Work out the finished part from the listing and answer in its coordinate system (mm). A direction names the side the tool comes from. Coordinates: 2 decimals unless noted, no trailing zeros. Loops run counter-clockwise (first coordinate to the right, second up) from the corner with the lowest first, then second, coordinate; pieces in that order, holes last. Notation, with made-up numbers: M 61,-24 L 89,-24 A19 ccw 89,-9 Z; hole C -8,50.5 d7. An arc over 180 degrees is marked long. Write each question's results on one line, items separated by ' | '.
```python
from build123d import *

# Parameters (mm, degrees)
F1_DEPTH = 63.5
F2_DEPTH = 12.7
F3_DEPTH = 25.4
F0_W     = 30.6498706341
F0_H     = 39.8745834827
F5_R     = 5.08


with BuildPart() as f1:
    # F0 (on Front) → F1 (new body, symmetric)
    with BuildSketch(Plane.XZ):
        Polygon((37.4401323497, 22.1690796316), (-51.7774410546, 22.1690796316), (-51.7774410546, -22.1690796316), (51.7774410546, -22.1690796316), (51.7774410546, 22.1690796316), align=None)
    extrude(amount=F1_DEPTH, both=True)

    # F0 (on Front) → F2 (join, symmetric)
    with BuildSketch(Plane.XZ):
        with BuildLine():
            Line((37.4401323497, 51.2318972406), (37.4401323497, 22.1690796316))
            Line((37.4401323497, 22.1690796316), (51.7774410546, 22.1690796316))
            Line((51.7774410546, 22.1690796316), (51.7774410546, 51.2318972406))
            ThreePointArc((51.7774410546, 51.2318972406), (57.0358954685, 63.9269292039), (69.7309274318, 69.1853836179))
            Line((69.7309274318, 69.1853836179), (80.344311893, 69.1853836179))
            Line((80.344311893, 69.1853836179), (80.344311893, 83.5226923227))
            Line((80.344311893, 83.5226923227), (69.7309274318, 83.5226923227))
            ThreePointArc((69.7309274318, 83.5226923227), (46.8978872594, 74.0649374131), (37.4401323497, 51.2318972406))
        make_face()
    extrude(amount=F2_DEPTH, both=True)

    # F0 (on Front) → F3 (join, symmetric)
    with BuildSketch(Plane.XZ):
        Polygon((80.344311893, 89.1226753592), (80.344311893, 83.5226923227), (80.344311893, 69.1853836179), (80.344311893, 49.2480918765), (110.9941825271, 49.2480918765), (110.9941825271, 89.1226753592), align=None)
    extrude(amount=F3_DEPTH, both=True)

    # F0 (on Front) → F4 (revolve)
    with BuildSketch(Plane.XZ):
        with Locations((126.3191178441, 69.1853836179)):
            Rectangle(F0_W, F0_H)
    revolve(axis=Axis((110.9941825271, 0, 69.1853836179), (0, 0, 1)))

    # F5
    f5_edges = [f1.edges().sort_by_distance(p)[0] for p in [
        (51.777441, 12.7, 36.700488),
        (46.897887, 12.7, 74.064937),
        (46.897887, -12.7, 74.064937),
        (80.344312, 25.4, 69.185384),
        (141.644053, 0, 89.122675),
        (87.092322, 25.4, 89.122675),
        (80.344312, 0, 89.122675),
        (87.092322, -25.4, 89.122675),
        (87.092322, 25.4, 49.248092),
        (141.644053, 0, 49.248092),
        (87.092322, -25.4, 49.248092),
        (80.344312, 0, 49.248092),
        (51.777441, -12.7, 36.700488),
        (57.035895, 12.7, 63.926929),
        (0, 63.5, 22.16908),
        (-51.777441, 0, 22.16908),
        (-51.777441, 63.5, 0),
        (-51.777441, 0, -22.16908),
        (0, 63.5, -22.16908),
        (51.777441, 38.1, 22.16908),
        (0, -63.5, 22.16908),
        (-51.777441, -63.5, 0),
        (51.777441, 63.5, 0),
        (0, -63.5, -22.16908),
        (51.777441, 0, -22.16908),
        (51.777441, -63.5, 0),
        (51.777441, -38.1, 22.16908),
    ]]
    fillet(f5_edges, radius=F5_R)


solid = f1.part
```
1) Given pin 1 Ø4 at (x, z) = (85.5, 76.5) entering from -Y; pin 2 Ø15.5 at (x, y) = (114.5, -2.5) entering from -Z; pin 3 Ø4 at (x, z) = (89.5, 64) entering from +Y; pin 4 Ø19 at (x, z) = (69.5, 48.5) entering from -Y, each flat-ended and moving along its own axis, determine where each tip first touches the part or whether it passes through.
Check result:
pin 1: y = -25.4 | pin 2: z = 49.25 | pin 3: y = 25.4 | pin 4: through
2) Find section C-C, the plane y = 0. Give the vertices of the cut face in (x, z).
Check result:
outline: M -51.78,-17.09 A5.08 ccw -46.7,-22.17 L 46.7,-22.17 A5.08 ccw 51.78,-17.09 L 51.78,51.23 A17.95 cw 69.73,69.19 L 80.34,69.19 L 80.34,54.33 A5.08 ccw 85.42,49.25 L 136.56,49.25 A5.08 ccw 141.64,54.33 L 141.64,84.04 A5.08 ccw 136.56,89.12 L 85.42,89.12 A5.08 ccw 80.34,84.04 L 80.34,83.52 L 69.73,83.52 A32.29 ccw 37.44,51.23 L 37.44,22.17 L -46.7,22.17 A5.08 ccw -51.78,17.09 Z
3) Which of the six approach directions +Z, -Z, +X, -X, +Y, -Y give full straight-line access (tool end or side, diameter ignored) to faces 1 (the face through (87, -25.4, 69)), 2 (the face through (75.11, -11.17, 70.63)), 3 (the face through (38.889, -11.172, 36.497)), 4 (the face through (75, 0, 69.185)), 5 (the face through (75, 0, 83.523))?
Check result:
face 1: +Z, -Z, -X, -Y | face 2: -Z, -Y | face 3: +Z, -X, -Y | face 4: -Z, +Y, -Y | face 5: +Z, -X, +Y, -Y
4) Find section B-B, the plane x = 90.5. Give the vertices of the cut face in (y, z), and give its area (3 significant figures).
Check result:
outline: M -25.4,54.33 A5.08 ccw -20.32,49.25 L 20.32,49.25 A5.08 ccw 25.4,54.33 L 25.4,84.04 A5.08 ccw 20.32,89.12 L -20.32,89.12 A5.08 ccw -25.4,84.04 Z | area: 2,000 mm^2
5) Find section A-A, the plane z = 36.5. Give the vertices of the cut face in (x, y).
Check result:
outline: M 37.44,-7.62 A5.08 ccw 42.52,-12.7 L 46.7,-12.7 A5.08 ccw 51.78,-7.62 L 51.78,7.62 A5.08 ccw 46.7,12.7 L 42.52,12.7 A5.08 ccw 37.44,7.62 Z
6) Straight lines are drawn through the part: probe 1 along X at (y, z) = (25, 11.5); probe 2 along Z at (x, y) = (-39.5, -58); probe 3 along X at (y, z) = (7, 34.5). For each, find the intervals that lie inside material, in ascending order. Write a range as [from, to].
Check result:
probe 1: [-51.78, 51.78] | probe 2: [-22.17, 22.17] | probe 3: [37.44, 51.78]
